Geometry check sheet. Reference: drawing and pictorial views, mm from the part's lowest x, y, z. A direction names the side the tool comes from. Round coordinates to 2 decimals unless told otherwise and drop trailing zeros. Write each loop counter-clockwise with the first axis right and the second up, starting at its lowest first coordinate (ties: lowest second). Pieces come first, ordered by that corner, then holes. Notation, with made-up numbers: (73.25, 41.25) - (128.25, 41.25) arc R21 cw to (128.25, 63.25) - close; hole circle Ø4 at (49.5, 55.25). An arc over 180 degrees is marked (long way). Use one line per item in the form item = value. Start each with the question number.
1) Scan lines: probe 1 along Z at (x, y) = (4, 3); probe 2 along Y at (x, z) = (6, 1); probe 3 along X at (y, z) = (1.5, 3) (1 decimal). Record each from-to range of solid material in increasing order.
2) Section check D-D (z = 7.25). Record the boundary of the cut face in (x, y), then the cut area to 3 significant figures.
3) Section check C-C (y = 1). Record the boundary of the cut face in (x, z).
4) Section check A-A (x = 4). Record the boundary of the cut face in (y, z).
5) Section check B-B (z = 4). Record the boundary of the cut face in (x, y).
6) Draft check along X on the marked faces 1, 2 and 3. Enter one of: +X half, -X half, draft (parallel to the pull), parting line (faces both ways), or undercut.
7) Gauge pin test, flat ends, axial feed: P1, Ø1, axis at y = 6.5, z = 5, coming from the +X side; P2, Ø4, axis at x = 4, z = 4, coming from the +Y side; P3, Ø3, axis at x = 33, z = 4, coming from the +Y side; P4, Ø2.5, axis at x = 14.5, y = 4, coming from the -Z side. Record the tip position at first contact, or that the pin passes through.
8) Set-up check for the marked faces 4, 5 and 6: record each of +Z, -Z, +X, -X, +Y, -Y from which the full face is reachable in a straight line by a thin tool's end or side.
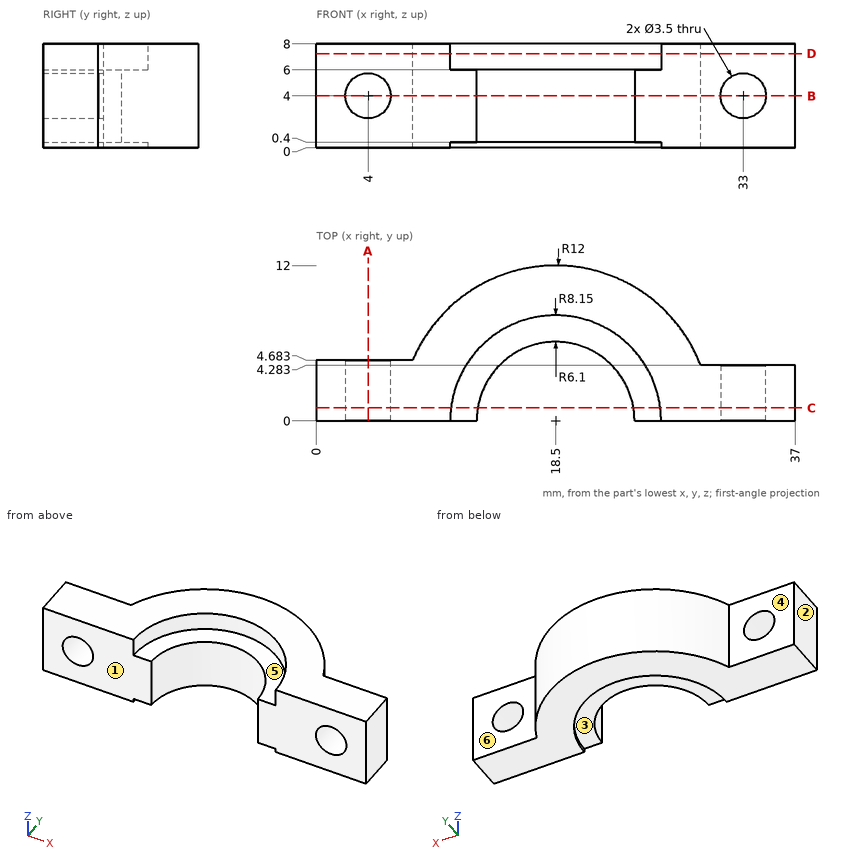
Results are:
q1.probe_1 = 0 to 2.25, 5.75 to 8
q1.probe_2 = 0 to 4.68
q1.probe_3 = 0 to 2.6, 5.4 to 12.6, 24.4 to 31.6, 34.4 to 37
q2.outline = (0, 0) - (10.35, 0) arc R8.15 cw to (26.65, 0) - (37, 0) - (37, 4.28) - (29.71, 4.28) arc R12 ccw to (7.45, 4.68) - (0, 4.68) - close
q2.area = 183 mm²
q3.outline = (0, 0) - (10.41, 0) - (10.41, 0.4) - (12.48, 0.4) - (12.48, 6) - (10.41, 6) - (10.41, 8) - (0, 8) - close; (24.52, 0.4) - (26.59, 0.4) - (26.59, 0) - (37, 0) - (37, 8) - (26.59, 8) - (26.59, 6) - (24.52, 6) - close; hole circle Ø3.5 at (4, 4); hole circle Ø3.5 at (33, 4)
q4.outline = (0, 0) - (4.68, 0) - (4.68, 2.25) - (0, 2.25) - close; (0, 5.75) - (4.68, 5.75) - (4.68, 8) - (0, 8) - close
q5.outline = (0, 0) - (2.25, 0) - (2.25, 4.68) - (0, 4.68) - close; (5.75, 0) - (12.4, 0) arc R6.1 cw to (24.6, 0) - (31.25, 0) - (31.25, 4.28) - (29.71, 4.28) arc R12 ccw to (7.45, 4.68) - (5.75, 4.68) - close; (34.75, 0) - (37, 0) - (37, 4.28) - (34.75, 4.28) - close
q6.face_1 = draft
q6.face_2 = -X half
q6.face_3 = undercut
q7.P1 = 28.89
q7.P2 = 4.68
q7.P3 = through
q7.P4 = 0.4
q8.face_4 = +Z, -Z, -X, +Y
q8.face_5 = +Z, -Y
q8.face_6 = +Z, -Z, +X, +Y
